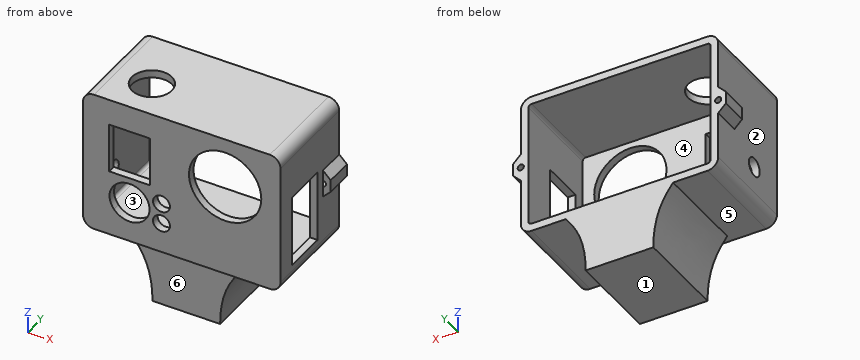
```python
from build123d import *

# Parameters (mm, degrees)
F1_DEPTH  = 30
F0_R      = 2.75
F0_W      = 13.2
F0_H      = 16.1
F0_R_2    = 11.75
F2_DEPTH  = 2.5
F3_R      = 6.5
F4_DEPTH  = 2.5
F5_R      = 3
F6_DEPTH  = 2.5
F7_W      = 14
F7_H      = 23.3
F8_DEPTH  = 2.5
F5_W      = 9
F5_H      = 9
F9_DEPTH  = 2.5
F7_W_2    = 9
F7_H_2    = 9
F10_DEPTH = 2.5
F11_SIZE  = 2.49999
F12_R     = 1
F13_DEPTH = 9


# Not quite as in the source:
# - a fillet or chamfer is up to 0.001 mm smaller than in the source, because OpenCascade refuses the exact size


with BuildPart() as f1:
    # F0 (on Front) → F1 (new body)
    with BuildSketch(Plane.XZ):
        with BuildLine():
            Line((-28.6, 20.6), (28.6, 20.6))
            ThreePointArc((28.6, 20.6), (29.3071067812, 20.3071067812), (29.6, 19.6))
            Line((29.6, 19.6), (29.6, -19.6))
            ThreePointArc((29.6, -19.6), (29.3071067812, -20.3071067812), (28.6, -20.6))
            Line((28.6, -20.6), (19.2463447419, -20.6))
            add(Edge.make_bspline(
                [(19.2463447419, -20.6), (18.6700440776, -21.4257741259), (18.043869698, -22.2429184725), (17.402758481, -23.1)],
                knots=[11.0100107819, 11.0100107819, 11.0100107819, 11.0100107819, 14.8362531821, 14.8362531821, 14.8362531821, 14.8362531821], degree=3))
            Line((17.402758481, -23.1), (28.6, -23.1))
            ThreePointArc((28.6, -23.1), (31.0748737342, -22.0748737342), (32.1, -19.6))
            Line((32.1, -19.6), (32.1, 19.6))
            ThreePointArc((32.1, 19.6), (31.0748737342, 22.0748737342), (28.6, 23.1))
            Line((28.6, 23.1), (-28.6, 23.1))
            ThreePointArc((-28.6, 23.1), (-31.0748737342, 22.0748737342), (-32.1, 19.6))
            Line((-32.1, 19.6), (-32.1, -19.6))
            ThreePointArc((-32.1, -19.6), (-31.0748737342, -22.0748737342), (-28.6, -23.1))
            Line((-28.6, -23.1), (-17.402758481, -23.1))
            add(Edge.make_bspline(
                [(-19.2463447419, -20.6), (-18.6700440776, -21.4257741259), (-18.043869698, -22.2429184725), (-17.402758481, -23.1)],
                knots=[11.0100107819, 11.0100107819, 11.0100107819, 11.0100107819, 14.8362531821, 14.8362531821, 14.8362531821, 14.8362531821], degree=3))
            Line((-19.2463447419, -20.6), (-28.6, -20.6))
            ThreePointArc((-28.6, -20.6), (-29.3071067812, -20.3071067812), (-29.6, -19.6))
            Line((-29.6, -19.6), (-29.6, 19.6))
            ThreePointArc((-29.6, 19.6), (-29.3071067812, 20.3071067812), (-28.6, 20.6))
        make_face()
        with BuildLine():
            add(Edge.make_bspline(
                [(19.2463447419, -20.6), (18.6700440776, -21.4257741259), (18.043869698, -22.2429184725), (17.402758481, -23.1)],
                knots=[11.0100107819, 11.0100107819, 11.0100107819, 11.0100107819, 14.8362531821, 14.8362531821, 14.8362531821, 14.8362531821], degree=3))
            Line((19.2463447419, -20.6), (-19.2463447419, -20.6))
            add(Edge.make_bspline(
                [(-19.2463447419, -20.6), (-18.6700440776, -21.4257741259), (-18.043869698, -22.2429184725), (-17.402758481, -23.1)],
                knots=[11.0100107819, 11.0100107819, 11.0100107819, 11.0100107819, 14.8362531821, 14.8362531821, 14.8362531821, 14.8362531821], degree=3))
            Line((-17.402758481, -23.1), (17.402758481, -23.1))
        make_face()
        with BuildLine():
            add(Edge.make_bspline(
                [(17.402758481, -23.1), (14.3686514172, -27.1562028058), (11, -32.1068893696), (11, -43.1)],
                knots=[14.8362531821, 14.8362531821, 14.8362531821, 14.8362531821, 32.9442331828, 32.9442331828, 32.9442331828, 32.9442331828], degree=3))
            Line((17.402758481, -23.1), (-17.402758481, -23.1))
            add(Edge.make_bspline(
                [(-17.402758481, -23.1), (-14.3686514172, -27.1562028058), (-11, -32.1068893696), (-11, -43.1)],
                knots=[14.8362531821, 14.8362531821, 14.8362531821, 14.8362531821, 32.9442331828, 32.9442331828, 32.9442331828, 32.9442331828], degree=3))
            Line((-11, -43.1), (11, -43.1))
        make_face()
    extrude(amount=-F1_DEPTH)

    # F0 (on Front) → F2 (join)
    with BuildSketch(Plane.XZ):
        with BuildLine():
            Line((-28.6, 20.6), (28.6, 20.6))
            ThreePointArc((28.6, 20.6), (29.3071067812, 20.3071067812), (29.6, 19.6))
            Line((29.6, 19.6), (29.6, -19.6))
            ThreePointArc((29.6, -19.6), (29.3071067812, -20.3071067812), (28.6, -20.6))
            Line((28.6, -20.6), (19.2463447419, -20.6))
            add(Edge.make_bspline(
                [(19.2463447419, -20.6), (18.6700440776, -21.4257741259), (18.043869698, -22.2429184725), (17.402758481, -23.1)],
                knots=[11.0100107819, 11.0100107819, 11.0100107819, 11.0100107819, 14.8362531821, 14.8362531821, 14.8362531821, 14.8362531821], degree=3))
            Line((17.402758481, -23.1), (28.6, -23.1))
            ThreePointArc((28.6, -23.1), (31.0748737342, -22.0748737342), (32.1, -19.6))
            Line((32.1, -19.6), (32.1, 19.6))
            ThreePointArc((32.1, 19.6), (31.0748737342, 22.0748737342), (28.6, 23.1))
            Line((28.6, 23.1), (-28.6, 23.1))
            ThreePointArc((-28.6, 23.1), (-31.0748737342, 22.0748737342), (-32.1, 19.6))
            Line((-32.1, 19.6), (-32.1, -19.6))
            ThreePointArc((-32.1, -19.6), (-31.0748737342, -22.0748737342), (-28.6, -23.1))
            Line((-28.6, -23.1), (-17.402758481, -23.1))
            add(Edge.make_bspline(
                [(-19.2463447419, -20.6), (-18.6700440776, -21.4257741259), (-18.043869698, -22.2429184725), (-17.402758481, -23.1)],
                knots=[11.0100107819, 11.0100107819, 11.0100107819, 11.0100107819, 14.8362531821, 14.8362531821, 14.8362531821, 14.8362531821], degree=3))
            Line((-19.2463447419, -20.6), (-28.6, -20.6))
            ThreePointArc((-28.6, -20.6), (-29.3071067812, -20.3071067812), (-29.6, -19.6))
            Line((-29.6, -19.6), (-29.6, 19.6))
            ThreePointArc((-29.6, 19.6), (-29.3071067812, 20.3071067812), (-28.6, 20.6))
        make_face()
        with BuildLine():
            ThreePointArc((29.6, 19.6), (29.3071067812, 20.3071067812), (28.6, 20.6))
            Line((28.6, 20.6), (-28.6, 20.6))
            ThreePointArc((-28.6, 20.6), (-29.3071067812, 20.3071067812), (-29.6, 19.6))
            Line((-29.6, 19.6), (-29.6, -19.6))
            ThreePointArc((-29.6, -19.6), (-29.3071067812, -20.3071067812), (-28.6, -20.6))
            Line((-28.6, -20.6), (-19.2463447419, -20.6))
            Line((-19.2463447419, -20.6), (19.2463447419, -20.6))
            Line((19.2463447419, -20.6), (28.6, -20.6))
            ThreePointArc((28.6, -20.6), (29.3071067812, -20.3071067812), (29.6, -19.6))
            Line((29.6, -19.6), (29.6, 19.6))
        make_face()
        with Locations((-6.6, -13.25)):
            Circle(F0_R, mode=Mode.SUBTRACT)
        with BuildLine():
            ThreePointArc((-10.5, -9.9), (-14.8124838728, -16.0208474244), (-22.027622521, -14.019831524))
            ThreePointArc((-22.027622521, -14.019831524), (-19.1875161272, -3.7791525756), (-10.5, -9.9))
        make_face(mode=Mode.SUBTRACT)
        with Locations((-17, 6.55)):
            Rectangle(F0_W, F0_H, mode=Mode.SUBTRACT)
        with Locations((-6.6, -6.55)):
            Circle(F0_R, mode=Mode.SUBTRACT)
        with Locations((14.1, 6.85)):
            Circle(F0_R_2, mode=Mode.SUBTRACT)
        with BuildLine():
            add(Edge.make_bspline(
                [(19.2463447419, -20.6), (18.6700440776, -21.4257741259), (18.043869698, -22.2429184725), (17.402758481, -23.1)],
                knots=[11.0100107819, 11.0100107819, 11.0100107819, 11.0100107819, 14.8362531821, 14.8362531821, 14.8362531821, 14.8362531821], degree=3))
            Line((19.2463447419, -20.6), (-19.2463447419, -20.6))
            add(Edge.make_bspline(
                [(-19.2463447419, -20.6), (-18.6700440776, -21.4257741259), (-18.043869698, -22.2429184725), (-17.402758481, -23.1)],
                knots=[11.0100107819, 11.0100107819, 11.0100107819, 11.0100107819, 14.8362531821, 14.8362531821, 14.8362531821, 14.8362531821], degree=3))
            Line((-17.402758481, -23.1), (17.402758481, -23.1))
        make_face()
    extrude(amount=F2_DEPTH)

    # F3 (on face) → F4 (cut, through all)
    with BuildSketch(Plane.XY.offset(23.1)):
        with Locations((-17.25, 10.3)):
            Circle(F3_R)
    extrude(amount=-F4_DEPTH, mode=Mode.SUBTRACT)

    # F5 (on face) → F6 (cut, through all)
    with BuildSketch(Plane(origin=(-32.1, 0, 0), x_dir=(0, -1, 0), z_dir=(-1, 0, 0))):
        with Locations((-10, -10.8)):
            Circle(F5_R)
    extrude(amount=-F6_DEPTH, mode=Mode.SUBTRACT)

    # F7 (on face) → F8 (cut, through all)
    with BuildSketch(Plane.YZ.offset(32.1)):
        with Locations((11, -5.95)):
            Rectangle(F7_W, F7_H)
    extrude(amount=-F8_DEPTH, mode=Mode.SUBTRACT)

    # F5 (on face) → F9 (join)
    with BuildSketch(Plane(origin=(-32.1, 0, 0), x_dir=(0, -1, 0), z_dir=(-1, 0, 0))):
        with Locations((-25.5, 0)):
            Rectangle(F5_W, F5_H)
    extrude(amount=F9_DEPTH)

    # F7 (on face) → F10 (join)
    with BuildSketch(Plane.YZ.offset(32.1)):
        with Locations((25.5, 0)):
            Rectangle(F7_W_2, F7_H_2)
    extrude(amount=F10_DEPTH)

    # F11 (size 2.5 in the source; OpenCascade refuses exactly that, so slightly less here)
    f11_edges = [f1.edges().sort_by_distance(p)[0] for p in [
        (-34.6, 25.5, -4.5),
        (-34.6, 25.5, 4.5),
        (34.6, 25.5, 4.5),
        (34.6, 25.5, -4.5),
    ]]
    chamfer(f11_edges, length=F11_SIZE)

    # F12 (on face) → F13 (cut)
    with BuildSketch(Plane(origin=(0, 30, 0), x_dir=(-1, 0, 0), z_dir=(0, 1, 0))):
        with Locations((-32.1, 0)):
            Circle(F12_R)
        with Locations((32.1, 0)):
            Circle(F12_R)
    extrude(amount=-F13_DEPTH, mode=Mode.SUBTRACT)


solid = f1.part
```
Input: part model. Units: mm. Frame: model coordinates. Face numbers are marked on the shaded views. A direction names the side the tool comes from. Give positions to 0.01 mm unless a question says otherwise; leave off trailing zeros. Write each loop counter-clockwise with the first axis right and the second up, starting at its lowest first coordinate (ties: lowest second). Pieces come first, ordered by that corner, then holes. Notation, with made-up numbers: (9, 4.25) - (68, 4.25) arc R30 cw to (68, 26.25) - close; hole circle Ø4 at (-6.5, -4.5). An arc over 180 degrees is marked (long way). Write item = value, one per line. Start each with the question number.
1) Cut plane A-A (x = -26). Return loops of the section in (y, z), and give its area (4 significant figures).
2) Cut plane B-B (z = 9.5). Return loops of the section in (x, y), and give its area (3 significant figures).
3) Material intervals for L1, parallel to Z at x = -17, y = -1; L2, parallel to Z at x = 5, y = 22; L3, parallel to X at y = 27, z = 0, sorted ascending. Write a range as [from, to].
4) Reachability of the marked faces 4, 5 and 6 from +Z, -Z, +X, -X, +Y, -Y: full face, straight path, thin tool, end or side. Return the list, or none.
5) Draft query along Z for the marked faces 1, 2 and 3. Return one class per face: pulls with the +Z half, pulls with the -Z half, needs draft (parallel to the pull), parting line crosses it, or undercut.
6) Cut plane C-C (y = 10.3). Give the number of separate pieces and of enclosed holes in the cut face, and give its area (3 significant figures).
7) Pin query (flat end, axial travel): pin 1 (5 mm diameter, centred on y = 6, z = 16, fed in from -X); pin 2 (1.2 mm diameter, centred on x = 31, y = 8.5, fed in from -Z); pin 3 (6 mm diameter, centred on x = -13, z = -13, fed in from +Y). Return the tip coordinate at first contact, or that it passes through.
Answers follow:
q1.outline = (-2.5, -23.1) - (30, -23.1) - (30, -20.6) - (0, -20.6) - (0, 20.6) - (30, 20.6) - (30, 23.1) - (-2.5, 23.1) - close
q1.area = 265.5 mm^2
q2.outline = (-32.1, -2.5) - (-23.6, -2.5) - (-23.6, 0) - (-29.6, 0) - (-29.6, 30) - (-32.1, 30) - close; (-10.4, -2.5) - (2.65, -2.5) - (2.65, 0) - (-10.4, 0) - close; (25.55, -2.5) - (32.1, -2.5) - (32.1, 30) - (29.6, 30) - (29.6, 0) - (25.55, 0) - close
q2.area = 220 mm^2
q3.L1 = [-23.1, -16.4], [-3.4, -1.5], [14.6, 23.1]
q3.L2 = [-43.1, -20.6], [20.6, 23.1]
q3.L3 = [-34.6, -33.1], [-31.1, -29.6], [29.6, 31.1], [33.1, 34.6]
q4.face_4 = +Y
q4.face_5 = -Z, -Y
q4.face_6 = -Z, +X, -X, -Y
q5.face_1 = pulls with the -Z half
q5.face_2 = needs draft
q5.face_3 = undercut
q6.separate_pieces = 3
q6.enclosed_holes = 0
q6.area = 927 mm^2
q7.pin_1 = -32.1
q7.pin_2 = -22.6
q7.pin_3 = 0
